from build123d import *

# Parameters (mm, degrees)
F1_DEPTH = 25


with BuildPart() as f1:
    # F0 (on Front) → F1 (new body)
    with BuildSketch(Plane.XZ):
        Polygon((2.144598, 50.810475), (-75.390868, 50.810475), (-75.390868, -13.692434), (2.144598, -13.692434), (2.144598, 21.116043), (48.665877, 21.116043), (48.665877, 50.810475), align=None)
    extrude(amount=F1_DEPTH)


solid = f1.part
For this review, take the finished solid that the model builds, in its own axes (mm). A direction names the side the tool comes from. Give positions to 0.01 mm unless a question says otherwise; leave off trailing zeros. Loops run counter-clockwise (first coordinate to the right, second up) from the corner with the lowest first, then second, coordinate; pieces in that order, holes last. Notation, with made-up numbers: M 14,-6 L 69,-6 A12 ccw 69,9 Z; hole C 14,75 d3. An arc over 180 degrees is marked long. Answer as a JSON object with one key per item and string values. Group by question number.
Q1. For probe 1 along Z at (x, y) = (15, -1.5); probe 2 along X at (y, z) = (-6, -2.5), list the stretches that pass through material, from the lowest coordinate up. Write a range as [from, to].
Q2. Insertion check: P1, Ø10, axis at x = -45.5, z = 22, coming from the +Y side; P2, Ø12.5, axis at y = -15.5, z = 0, coming from the +X side. Each pin has a flat end and moves straight along its axis. Give the tip position at first contact, or say it passes through.
Q3. Tool access review of faces 1 (the flat face through (-28, 0, 19)), 2 (the flat face through (25, -12, 21.116)): name each direction out of +Z, -Z, +X, -X, +Y, -Y from which nothing blocks a thin tool from reaching the whole face with its end or side.
Q4. Add section A-A on y = -13. Give the boundary of the cut face in (x, z).
Q5. Add section B-B on x = 35. Give the boundary of the cut face in (y, z), and give its area (3 significant figures).
Q6. Add section C-C on z = 13.5. Give the boundary of the cut face in (x, y).
Checked values:
{
 "1": {"probe 1": "[21.12, 50.81]", "probe 2": "[-75.39, 2.14]"},
 "2": {"P1": "y = 0", "P2": "x = 2.14"},
 "3": {"face 1": "+Z, -Z, +X, -X, +Y", "face 2": "-Z, +X, +Y, -Y"},
 "4": {"outline": "M -75.39,-13.69 L 2.14,-13.69 L 2.14,21.12 L 48.67,21.12 L 48.67,50.81 L -75.39,50.81 Z"},
 "5": {"outline": "M -25,21.12 L 0,21.12 L 0,50.81 L -25,50.81 Z", "area": "742 mm²"},
 "6": {"outline": "M -75.39,-25 L 2.14,-25 L 2.14,0 L -75.39,0 Z"}
}
